Could you check a few things on this model? Use its own coordinates, in mm. Face numbers are marked on the shaded views. Round coordinates to 2 decimals unless told otherwise and drop trailing zeros. Order: outer loops, then holes, each group sorted by start corner. A loop starts at its lowest first (then second) coordinate and runs counter-clockwise, first axis right, second up. Notation, with made-up numbers: (-1.5, -13) -> (12.5, -13) arc R18 cw to (12.5, -7) -> close; hole circle Ø10 at (-5, 13.25). An arc over 180 degrees is marked (long way). Put each result on its own line as item: value. Start each with the question number.
Autodesk Inventor part; units mm, degrees
ref_plane "YZ Plane" through (0, 0, 0) normal (1, 0, 0) x (0, 1, 0)
ref_plane "XZ Plane" through (0, 0, 0) normal (0, 1, 0) x (-1, 0, 0)
ref_plane "XY Plane" through (0, 0, 0) normal (0, 0, 1) x (1, 0, 0)
sketch "Boceto principal" plane through (0, 0, 0) normal (1, 0, 0) x (0, 1, 0)
  line L0 (0, -1) -> (0, -3)
  line L1 (0, -3) -> (2, -3)
  line L2 (2, -3) -> (2, -2)
  line L3 (2, -2) -> (6, -2)
  line L4 (7, -3) -> (7, -27)
  line L5 (6, -28) -> (2, -28)
  line L6 (2, -28) -> (2, -27)
  line L7 (2, -27) -> (0, -27)
  line L8 (0, -27) -> (0, -29)
  line L9 (1, -30) -> (8, -30)
  line L10 (9, -29) -> (9, -1)
  line L11 (8, 0) -> (1, 0)
  arc A0 (1, 0) -> (0, -1) centre (1, -1) ccw
  arc A1 (7, -3) -> (6, -2) centre (6, -3) ccw
  arc A2 (6, -28) -> (7, -27) centre (6, -27) ccw
  arc A3 (0, -29) -> (1, -30) centre (1, -29) ccw
  arc A4 (8, -30) -> (9, -29) centre (8, -29) ccw
  arc A5 (9, -1) -> (8, 0) centre (8, -1) ccw
extrude "Extrusion1" add sketch "Boceto principal" along normal blind 317
sketch "Boceto esquinas" plane through (0, 0, 0) normal (0, 1, 0) x (-1, 0, 0)
  line L0 (0, 0) -> (-30, 0)
  line L1 (-30, 0) -> (0, -30)
  line L2 (0, -30) -> (0, 0)
  line L3 (-287, 0) -> (-317, 0)
  line L4 (-317, 0) -> (-317, -30)
  line L5 (-317, -30) -> (-287, 0)
extrude "Extrusion2" cut sketch "Boceto esquinas" along normal blind 10
properties part number "Tapa 30x30 317mm" material "PVC, Flexible"
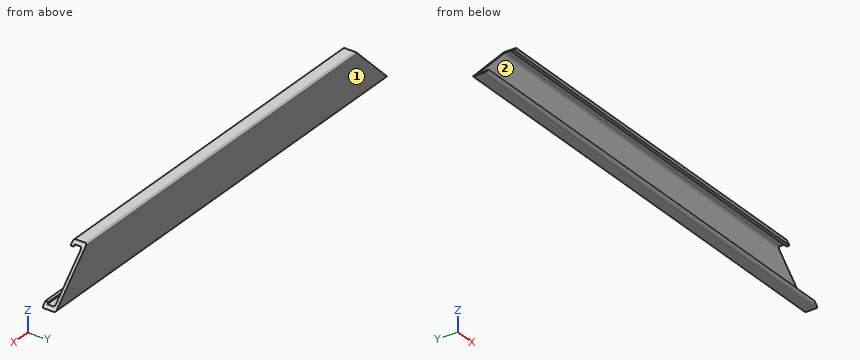
1. Thinking about a two-plate mould opening in Z: for the marked faces 1 and 2, which applies, +Z half, -Z half, draft (parallel to the pull), parting line (faces both ways), or undercut?
2. If we section it at C-C, the plane z = -20.5: Please give me the cut outline in (x, y), then the cut area to 3 significant figures.
3. If we section it at B-B, the plane z = -7: Please give me the cut outline in (x, y), then the cut area to 3 significant figures.
4. I need wall thicknesses on L1, parallel to Z at x = 211, y = 4.25; L2, parallel to Z at x = 152, y = 1; L3, parallel to Y at x = 187, z = -5.5. Which ranges of each line are inside material? Lowest first, please.
5. If we section it at A-A, the plane x = 266.5: Please give me the cut outline in (y, z), then the cut area to 3 significant figures.
6. For pin 1 Ø5 at (y, z) = (6.5, -6) entering from +X; pin 2 Ø12 at (x, z) = (126.5, -20.5) entering from -Y, each with a flat end and sliding along its axis, tell me the tip position at first contact or that it passes through.
Results below:
1. face 1: draft
1. face 2: undercut
2. outline: (9.5, 7) -> (307.5, 7) -> (307.5, 9) -> (9.5, 9) -> close
2. area: 596 mm2
3. outline: (23, 7) -> (294, 7) -> (294, 9) -> (23, 9) -> close
3. area: 542 mm2
4. L1: -30 to -28, -2 to 0
4. L2: -30 to -27, -3 to 0
4. L3: 7 to 9
5. outline: (0, -29) arc R1 ccw to (1, -30) -> (8, -30) arc R1 ccw to (9, -29) -> (9, -1) arc R1 ccw to (8, 0) -> (1, 0) arc R1 ccw to (0, -1) -> (0, -3) -> (2, -3) -> (2, -2) -> (6, -2) arc R1 cw to (7, -3) -> (7, -27) arc R1 cw to (6, -28) -> (2, -28) -> (2, -27) -> (0, -27) -> close
5. area: 91.6 mm2
6. pin 1: x = 295.45
6. pin 2: y = 7
